Source: CAD feature listing. Evaluate the final solid. Frame: model axes, mm. A direction names the side the tool comes from. Give positions to 0.01 mm unless a question says otherwise; leave off trailing zeros. Write each loop counter-clockwise with the first axis right and the second up, starting at its lowest first coordinate (ties: lowest second). Pieces come first, ordered by that corner, then holes.
```python
from build123d import *

# Parameters (mm, degrees)
SKETCH_1_W          = 75
SKETCH_1_H          = 40
EXTRUDE_1_DEPTH     = 60
SKETCH_2_R          = 19
EXTRUDE_2_DEPTH     = 75
SKETCH_3_W          = 36.2897677
SKETCH_3_H          = 40
EXTRUDE_3_DEPTH     = 780
SKETCH_7_R          = 15
CUT_EXTRUDE_1_DEPTH = 800


with BuildPart() as part:
    # 草圖1 → 填料-伸長1 (new body)
    with BuildSketch(Plane.XY):
        with Locations((-6.874209628, -1.106382979)):
            Rectangle(SKETCH_1_W, SKETCH_1_H)
    extrude(amount=EXTRUDE_1_DEPTH)

    # 草圖2 → 填料-伸長2 (add)
    with BuildSketch(Plane.XY.offset(60)):
        with Locations((11.625790372, -1.025700825)):
            Circle(SKETCH_2_R)
    extrude(amount=EXTRUDE_2_DEPTH)

    # 草圖3 → 填料-伸長3 (add)
    with BuildSketch(Plane.XY.offset(60)):
        with Locations((-26.229325778, -1.106382979)):
            Rectangle(SKETCH_3_W, SKETCH_3_H)
    extrude(amount=EXTRUDE_3_DEPTH)

    # 草圖7 → 除料-伸長1 (cut)
    with BuildSketch(Plane.XY.offset(840)):
        with Locations((-26.229325778, -1.106382979)):
            Circle(SKETCH_7_R)
    extrude(amount=-CUT_EXTRUDE_1_DEPTH, mode=Mode.SUBTRACT)


solid = part.part
```
1. Cut plane A-A, the plane z = 95. Return the cut outline in (x, y), then the cut area to 3 significant figures.
2. Contact query for flat-ended pins moving along their axis: P1, Ø8, axis at y = 13.5, z = 512.5, coming from the +X side; P2, Ø3, axis at x = 3, y = -7.5, coming from the +Z side; P3, Ø15, axis at x = -27.5, y = -5, coming from the +Z side. Output: stop coordinate, or through.
3. Cut plane C-C, the plane y = 6. Return the cut outline in (x, z).
4. Cut plane D-D, the plane z = 658.5. Return the cut outline in (x, y).
5. Cut plane B-B, the plane x = -28.5. Return the cut outline in (y, z).
6. Access query for faces 1 (the flat face through (-7, -1, 0)), 2 (the flat face through (-26, -1, 40)). Directions: +Z, -Z, +X, -X, +Y, -Y. A direction counts if a zero-diameter tool reaches every point of the face in a straight line with its end or side. Return the directions, or none.
7. Mould query, pull axis X, two halves, no side actions, for faces 3 (the flat face through (11, -1, 135)), 4 (the flat face through (30.626, -1, 30)), 5 (the flat face through (-7.5, 1.9, 60)). Classes: +X half, -X half, draft (parallel to the pull), parting line (faces both ways), or undercut.
8. Line query: L1, parallel to X at y = -2.5, z = 136.5; L2, parallel to X at y = -1, z = 48; L3, parallel to Y at x = -27.5, z = 469.5. Output: solid intervals per line, ascending.
Response values:
1. outline: (-44.37, -21.11) - (-8.08, -21.11) - (-8.08, 18.89) - (-44.37, 18.89) - close; circle Ø38 at (11.63, -1.03); hole circle Ø30 at (-26.23, -1.11)
1. area: 1,880 mm2
2. P1: stops at x = -8.08
2. P2: stops at z = 135
2. P3: stops at z = 40
3. outline: (-44.37, 0) - (30.63, 0) - (30.63, 60) - (29.28, 60) - (29.28, 135) - (-6.03, 135) - (-6.03, 60) - (-8.08, 60) - (-8.08, 840) - (-13.02, 840) - (-13.02, 40) - (-39.44, 40) - (-39.44, 840) - (-44.37, 840) - close
4. outline: (-44.37, -21.11) - (-8.08, -21.11) - (-8.08, 18.89) - (-44.37, 18.89) - close; hole circle Ø30 at (-26.23, -1.11)
5. outline: (-21.11, 0) - (18.89, 0) - (18.89, 840) - (13.72, 840) - (13.72, 40) - (-15.93, 40) - (-15.93, 840) - (-21.11, 840) - close
6. face 1: -Z, +X, -X, +Y, -Y
6. face 2: +Z
7. face 3: draft
7. face 4: +X half
7. face 5: undercut
8. L1: x = -44.37 to -41.16, -11.29 to -8.08
8. L2: x = -44.37 to -41.23, -11.23 to 30.63
8. L3: y = -21.11 to -16.05, 13.84 to 18.89
